from build123d import *

# Parameters (mm, degrees)
F1_DEPTH  = 63.5
F2_DEPTH  = 25.4
F3_DEPTH  = 7.9375
F4_R      = 6.35
F2_FACE_W = 50.8
F2_FACE_H = 19.05
F5_DEPTH  = 25.4


with BuildPart() as f1:
    # F0 (on Front) → F1 (new body, symmetric)
    with BuildSketch(Plane.XZ):
        Polygon((22.225, 9.525), (-41.275, 9.525), (-41.275, -9.525), (41.275, -9.525), (41.275, 9.525), align=None)
    extrude(amount=F1_DEPTH, both=True)

    # F0 (on Front) → F2 (join, symmetric)
    with BuildSketch(Plane.XZ):
        with BuildLine():
            Line((22.225, 27.602186), (22.225, 9.525))
            Line((22.225, 9.525), (41.275, 9.525))
            Line((41.275, 9.525), (41.275, 27.602186))
            ThreePointArc((41.275, 27.602186), (44.485924, 37.174898), (52.819795, 42.8752))
            Line((52.819795, 42.8752), (60.325, 42.8752))
            Line((60.325, 42.8752), (60.325, 61.9252))
            Line((60.325, 61.9252), (50.693503, 61.9252))
            ThreePointArc((50.693503, 61.9252), (30.268326, 49.898626), (22.225, 27.602186))
        make_face()
    extrude(amount=F2_DEPTH, both=True)

    # F0 (on Front) → F3 (join, symmetric)
    with BuildSketch(Plane.XZ):
        with BuildLine():
            add(Edge.make_bspline(
                [(-41.275, 9.525), (-41.602355, 48.730145), (13.809814, 60.34423), (50.693503, 61.9252)],
                knots=[0, 0, 0, 0, 105.848885, 105.848885, 105.848885, 105.848885], degree=3))
            Line((-41.275, 9.525), (22.225, 9.525))
            Line((22.225, 9.525), (22.225, 27.602186))
            ThreePointArc((22.225, 27.602186), (30.268326, 49.898626), (50.693503, 61.9252))
        make_face()
    extrude(amount=F3_DEPTH, both=True)

    # F4
    f4_edges = [f1.edges().sort_by_distance(p)[0] for p in [
        (41.275, -63.5, 0),
        (-41.275, -63.5, 0),
        (41.275, 63.5, 0),
        (-41.275, 63.5, 0),
    ]]
    fillet(f4_edges, radius=F4_R)

    # F2_face (on face) → F5 (join)
    with BuildSketch(Plane(origin=(60.325, 0, 52.4002), x_dir=(0, 1, 0), z_dir=(1, 0, 0))):
        Rectangle(F2_FACE_W, F2_FACE_H)
    extrude(amount=F5_DEPTH)

    # F0 (on Front) → F6 (revolve)
    with BuildSketch(Plane.XZ):
        Polygon((85.725, 66.675), (85.725, 61.9252), (85.725, 42.8752), (85.725, 38.1), (111.125, 38.1), (111.125, 66.675), align=None)
    revolve(axis=Axis((85.725, 0, 52.3875), (0, 0, -1)))


solid = f1.part
Geometry check sheet. Reference: the model listing, model coordinates, mm. A direction names the side the tool comes from. Give positions to 0.01 mm unless a question says otherwise; leave off trailing zeros. Order: outer loops, then holes, each group sorted by start corner. A loop starts at its lowest first (then second) coordinate and runs counter-clockwise, first axis right, second up.
1. Draft check along X on faces 4 (the face through (-5, -7.938, 30)), 5 (the face through (58, 0, 42.875)), 6 (the face through (22.225, -17, 19)). Enter one of: pulls with the +X half, pulls with the -X half, needs draft (parallel to the pull), parting line crosses it, or undercut.
Completed:
face 4: needs draft
face 5: undercut
face 6: pulls with the -X half
2. Scan lines: line 1 (X direction, y = -13, z = 3) (3 decimals); line 2 (Z direction, x = -31.5, y = -36.5) (3 decimals); line 3 (Y direction, x = 26.5, z = 51). Record each from-to range of solid material in increasing order.
Completed:
line 1: x = -41.275 to 41.275
line 2: z = -9.525 to 9.525
line 3: y = -7.94 to 7.94
3. Depth check by flat-ended pin: pin 1 (1.5 mm diameter, centred on x = 35, z = 22.5, fed in from -Y); pin 2 (16.5 mm diameter, centred on x = -13.5, y = 31.5, fed in from +Z) (3 decimals); pin 3 (12 mm diameter, centred on y = 9.5, z = 17.5, fed in from +X) (3 decimals); pin 4 (1.5 mm diameter, centred on y = 28.5, z = 11, fed in from +X). Enter the tip coordinate at first touch or a pass-through.
Completed:
pin 1: stops at y = -25.4
pin 2: stops at z = 9.525
pin 3: stops at x = 41.275
pin 4: passes through
4. Access from +Z, -Z, +X, -X, +Y, -Y to the whole of each face (thin tool, end or side, straight path). Record for faces 1 (the face through (86, 0, 38.1)), 2 (the face through (-5, 7.938, 30)), 3 (the face through (30.486, -16.791, 50.158)).
Completed:
face 1: -Z, +X, +Y, -Y
face 2: +Z, -X, +Y
face 3: +Z, -X, -Y
5. Sectioned sample at A-A (x = 71). Record the boundary of the cut face in (y, z) (3 decimals), then the cut area to 3 significant figures.
Completed:
outline: (-25.4, 42.875) - (-20.696, 42.875) - (-20.696, 38.1) - (20.696, 38.1) - (20.696, 42.875) - (25.4, 42.875) - (25.4, 61.925) - (20.696, 61.925) - (20.696, 66.675) - (-20.696, 66.675) - (-20.696, 61.925) - (-25.4, 61.925) - close
area: 1,360 mm2
6. Sectioned sample at D-D (y = -37). Record the boundary of the cut face in (x, z) (3 decimals).
Completed:
outline: (-41.275, -9.525) - (41.275, -9.525) - (41.275, 9.525) - (-41.275, 9.525) - close
